from build123d import *

# Parameters (mm, degrees)
SKETCH1_W           = 17
SKETCH1_H           = 17
BOSS_EXTRUDE1_DEPTH = 1156.4
CUT_EXTRUDE4_START  = -20
SKETCH5_W           = 14
SKETCH5_H           = 40
CUT_EXTRUDE4_DEPTH  = 10
CUT_EXTRUDE5_DEPTH  = 1157.745849355


with BuildPart() as part:
    # Sketch1 → Boss-Extrude1 (new body)
    with BuildSketch(Plane(origin=(0, 0, 0), x_dir=(1, 0, 0), z_dir=(0, 1, 0))):
        with BuildLine():
            Line((0.5, 0), (19.5, 0))
            ThreePointArc((19.5, 0), (19.853553391, 0.146446609), (20, 0.5))
            Line((20, 0.5), (20, 19.5))
            ThreePointArc((20, 19.5), (19.853553391, 19.853553391), (19.5, 20))
            Line((19.5, 20), (0.5, 20))
            ThreePointArc((0.5, 20), (0.146446609, 19.853553391), (0, 19.5))
            Line((0, 19.5), (0, 0.5))
            ThreePointArc((0, 0.5), (0.146446609, 0.146446609), (0.5, 0))
        make_face()
        with Locations((10, 10)):
            Rectangle(SKETCH1_W, SKETCH1_H, mode=Mode.SUBTRACT)
    extrude(amount=BOSS_EXTRUDE1_DEPTH)

    # Sketch5 → Cut-Extrude4 (cut)
    with BuildSketch(Plane.ZY.offset(CUT_EXTRUDE4_START)):
        with Locations((-10, 1136.4)):
            Rectangle(SKETCH5_W, SKETCH5_H)
    cut_extrude4 = extrude(amount=CUT_EXTRUDE4_DEPTH, mode=Mode.SUBTRACT)

    # Sketch6 → Cut-Extrude5 (cut, through all)
    with BuildSketch(Plane(origin=(0, 0, -20), x_dir=(-1, 0, 0), z_dir=(0, 0, -1))):
        Polygon((-15, 1156.4), (-15, 1153.4), (-3, 1146.4), (0, 1146.4), (0, 1156.4), align=None)
    cut_extrude5 = extrude(amount=-CUT_EXTRUDE5_DEPTH, mode=Mode.SUBTRACT)

    # Mirror1: Cut-Extrude4, Cut-Extrude5 across plane
    add(cut_extrude4.mirror(Plane.ZX.offset(578.2)), mode=Mode.SUBTRACT)
    add(cut_extrude5.mirror(Plane.ZX.offset(578.2)), mode=Mode.SUBTRACT)


solid = part.part
Source: CAD feature listing. Evaluate the final solid. Frame: model axes, mm. Coordinates: 2 decimals unless noted, no trailing zeros. Order: outer loops, then holes, each group sorted by start corner. A loop starts at its lowest first (then second) coordinate and runs counter-clockwise, first axis right, second up. Notation, with made-up numbers: M 79.25,53 L 89.25,53 A13 cw 89.25,69 Z; hole C 88.25,71 d3. An arc over 180 degrees is marked long. Write each question's results on one line, items separated by ' | '. Start each with the question number.
1. Material intervals for L1, parallel to X at y = 109.5, z = -14.5; L2, parallel to Z at x = 15.5, y = 701.5; L3, parallel to Y at x = 18.75, z = -4, sorted ascending.
2. Section C-C, the plane y = 70. Return the cut outline in (x, z), then the cut area to 3 significant figures.
3. Section B-B, the plane x = 7. Return the cut outline in (y, z), then the cut area to 3 significant figures.
4. Pin query (flat end, axial travel): pin 1 (1.5 mm diameter, centred on x = 1.5, z = -8.5, fed in from -Y); pin 2 (1.6 mm diameter, centred on y = 2, z = -19.5, fed in from -X); pin 3 (1.6 mm diameter, centred on x = 19, z = -13, fed in from -Y). Return the tip coordinate at first contact, or that it passes through.
5. Section A-A, the plane z = -9.5. Return the cut outline in (x, y), then the cut area to 3 significant figures.
Solution:
1) L1: 0 to 1.5, 18.5 to 20 | L2: -20 to -18.5, -1.5 to 0 | L3: 40 to 1116.4
2) outline: M 0,-19.5 A0.5 ccw 0.5,-20 L 19.5,-20 A0.5 ccw 20,-19.5 L 20,-0.5 A0.5 ccw 19.5,0 L 0.5,0 A0.5 ccw 0,-0.5 Z; hole M 1.5,-18.5 L 18.5,-18.5 L 18.5,-1.5 L 1.5,-1.5 Z | area: 111 mm²
3) outline: M 7.67,-20 L 1148.73,-20 L 1148.73,-18.5 L 7.67,-18.5 Z; M 7.67,-1.5 L 1148.73,-1.5 L 1148.73,0 L 7.67,0 Z | area: 3,420 mm²
4) pin 1: y = 10 | pin 2: x = 15 | pin 3: y = 40
5) outline: M 0,10 L 1.5,10 L 1.5,1146.4 L 0,1146.4 Z; M 18.5,40 L 20,40 L 20,1116.4 L 18.5,1116.4 Z | area: 3,320 mm²
